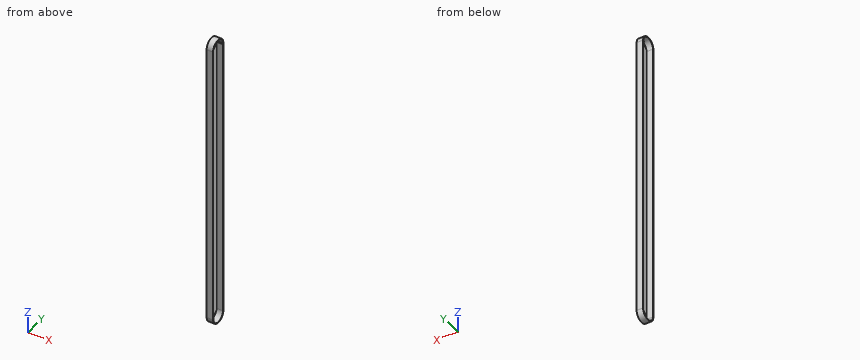
from build123d import *

# Parameters (mm, degrees)
BOSS_EXTRUDE1_DEPTH = 6
BOSS_EXTRUDE2_DEPTH = 6


with BuildPart() as part:
    # Sketch1 → Boss-Extrude1 (new body)
    with BuildSketch(Plane(origin=(0, 0, 0), x_dir=(0, 0, -1), z_dir=(1, 0, 0))):
        with BuildLine():
            Line((0, 7.3), (262, 7.3))
            ThreePointArc((262, 7.3), (269.3, 0), (262, -7.3))
            Line((262, -7.3), (0, -7.3))
            ThreePointArc((0, -7.3), (-7.3, 0), (0, 7.3))
        make_face()
        with BuildLine():
            Line((0, 6.7), (262, 6.7))
            ThreePointArc((262, 6.7), (268.7, 0), (262, -6.7))
            Line((262, -6.7), (0, -6.7))
            ThreePointArc((0, -6.7), (-6.7, 0), (0, 6.7))
        make_face(mode=Mode.SUBTRACT)
    extrude(amount=BOSS_EXTRUDE1_DEPTH)

    # Sketch2 → Boss-Extrude2 (add, through all)
    with BuildSketch(Plane(origin=(0, 0, 0), x_dir=(0, 0, -1), z_dir=(1, 0, 0))):
        with BuildLine():
            Line((0.187938524, 6.568404029), (0.346923655, 6.131595971))
            ThreePointArc((0.346923655, 6.131595971), (0.420146892, 6.036169591), (0.534862179, 6))
            Line((0.534862179, 6), (1.158985131, 6))
            ThreePointArc((1.158985131, 6), (1.273700418, 6.036169591), (1.346923655, 6.131595971))
            Line((1.346923655, 6.131595971), (1.505908786, 6.568404029))
            ThreePointArc((1.505908786, 6.568404029), (1.579132023, 6.663830409), (1.69384731, 6.7))
            Line((1.69384731, 6.7), (0, 6.7))
            ThreePointArc((0, 6.7), (0.114715287, 6.663830409), (0.187938524, 6.568404029))
        make_face()
    extrude(amount=BOSS_EXTRUDE2_DEPTH)


solid = part.part
For this review, take the finished solid that the model builds, in its own axes (mm). Round coordinates to 2 decimals unless told otherwise and drop trailing zeros. Order: outer loops, then holes, each group sorted by start corner. A loop starts at its lowest first (then second) coordinate and runs counter-clockwise, first axis right, second up. Notation, with made-up numbers: M 76.25,-16.75 L 96.25,-16.75 A18 cw 96.25,1.25 Z; hole C -16.5,32.5 d7. An arc over 180 degrees is marked long. Use a Markdown table: item, result. Add a question column.
Item 1: Add section C-C, the plane z = -21. Give the boundary of the cut face in (x, y), then the cut area to 3 significant figures.
Item 2: Add section B-B, the plane x = 3.15. Give the boundary of the cut face in (y, z), then the cut area to 3 significant figures.
Item 3: Add section A-A, the plane y = 0. Give the boundary of the cut face in (x, z).
Item 4: To check wall thickness, follow line 1 along Y through (x, z) = (2.7, -166.5); line 2 along Z through (x, y) = (4.7, -0.5); line 3 along Z through (x, y) = (0.75, 3.75). State the ranges of each line that lie inside material, in increasing order.
Geometry results:
| question | item | result |
|---|---|---|
| 1 | outline | M 0,-7.3 L 6,-7.3 L 6,-6.7 L 0,-6.7 Z; M 0,6.7 L 6,6.7 L 6,7.3 L 0,7.3 Z |
| 1 | area | 7.20 mm² |
| 2 | outline | M -7.3,-262 A7.3 ccw 7.3,-262 L 7.3,0 A7.3 ccw -7.3,0 Z; hole M -6.7,-262 A6.7 ccw 6.7,-262 L 6.7,-1.69 A0.2 ccw 6.57,-1.51 L 6.13,-1.35 A0.2 cw 6,-1.16 L 6,-0.53 A0.2 cw 6.13,-0.35 L 6.57,-0.19 A0.2 ccw 6.7,0 A6.7 ccw -6.7,0 Z |
| 2 | area | 342 mm² |
| 3 | outline | M 0,-269.3 L 6,-269.3 L 6,-268.7 L 0,-268.7 Z; M 0,6.7 L 6,6.7 L 6,7.3 L 0,7.3 Z |
| 4 | line 1 | y = -7.3 to -6.7, 6.7 to 7.3 |
| 4 | line 2 | z = -269.28 to -268.68, 6.68 to 7.28 |
| 4 | line 3 | z = -268.26 to -267.55, 5.55 to 6.26 |
